Build history of the part. All positions in model axes, mm. Face numbers are marked on the shaded views. Round coordinates to 2 decimals unless told otherwise and drop trailing zeros. Write each loop counter-clockwise with the first axis right and the second up, starting at its lowest first coordinate (ties: lowest second). Pieces come first, ordered by that corner, then holes. Notation, with made-up numbers: (73.25, -4) - (107.25, -4) arc R29 cw to (107.25, 20) - close; hole circle Ø7 at (-7, 19.5). An arc over 180 degrees is marked (long way). Write each question's results on one line, items separated by ' | '.
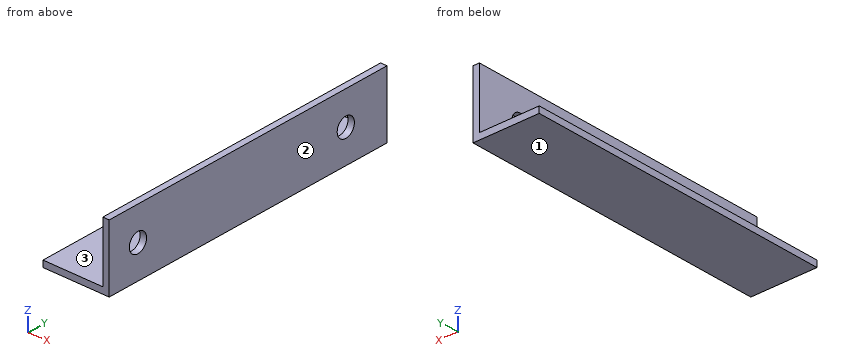
from build123d import *

# Parameters (mm, degrees)
F4_DEPTH = 145
F5_R     = 4.5
F6_DEPTH = 3


with BuildPart() as f4:
    # F3 (on Front) → F4 (new body)
    with BuildSketch(Plane.XZ):
        Polygon((-31, 0), (0, 0), (0, 31), (-3, 31), (-3, 3), (-31, 3), align=None)
    extrude(amount=F4_DEPTH)

    # F5 (on face) → F6 (cut, through all)
    with BuildSketch(Plane.YZ):
        with Locations((-130, 15.5)):
            Circle(F5_R)
        with Locations((-21.5, 15.5)):
            Circle(F5_R)
    extrude(amount=-F6_DEPTH, mode=Mode.SUBTRACT)


solid = f4.part
(1) Slice it at A-A, the plane z = 15.5. Write the cut outline in (x, y), and give its area (3 significant figures).
Worked answers:
outline: (-3, -145) - (0, -145) - (0, -134.5) - (-3, -134.5) - close; (-3, -125.5) - (0, -125.5) - (0, -26) - (-3, -26) - close; (-3, -17) - (0, -17) - (0, 0) - (-3, 0) - close | area: 381 mm2
(2) Flat gauge pins, fed straight in: pin 1 Ø14 at (x, y) = (-18, -85.5) entering from +Z; pin 2 Ø10 at (y, z) = (-103.5, 18.5) entering from -X. Where does each tip first touch, or does it go through?
Worked answers:
pin 1: stops at z = 3 | pin 2: stops at x = -3
(3) Slice it at D-D, the plane x = -19. Write the cut outline in (y, z).
Worked answers:
outline: (-145, 0) - (0, 0) - (0, 3) - (-145, 3) - close
(4) Drill centre lines: probe 1 along Y at (x, z) = (-2, 15); probe 2 along Z at (x, y) = (-1, -21); probe 3 along X at (y, z) = (-86, 14.5). Where is each one in solid material? Low to high. Write a range as [from, to].
Worked answers:
probe 1: y = [-145, -134.47], [-125.53, -25.97], [-17.03, 0] | probe 2: z = [0, 11.03], [19.97, 31] | probe 3: x = [-3, 0]
(5) Slice it at B-B, the plane y = -130. Write the cut outline in (x, z).
Worked answers:
outline: (-31, 0) - (0, 0) - (0, 11) - (-3, 11) - (-3, 3) - (-31, 3) - close; (-3, 20) - (0, 20) - (0, 31) - (-3, 31) - close
(6) Slice it at C-C, the plane y = -47. Write the cut outline in (x, z).
Worked answers:
outline: (-31, 0) - (0, 0) - (0, 31) - (-3, 31) - (-3, 3) - (-31, 3) - close
(7) Two-plate mould, pull along Z, no slides. Class the marked faces 1, 2 and 3: released by +Z, released by -Z, zero draft, split by the parting line, or undercut.
Worked answers:
face 1: released by -Z | face 2: zero draft | face 3: released by +Z
